Check sheet for the modelled part. Datum: model origin and axes. Units: mm. Face numbers are marked on the shaded views. A direction names the side the tool comes from. Round coordinates to 2 decimals unless told otherwise and drop trailing zeros. Order: outer loops, then holes, each group sorted by start corner. A loop starts at its lowest first (then second) coordinate and runs counter-clockwise, first axis right, second up.
Q1. Scan lines: probe 1 along X at (y, z) = (100, -7.5); probe 2 along X at (y, z) = (34, 19); probe 3 along Z at (x, y) = (-6, 18.5). Record each from-to range of solid material in increasing order.
Q2. Depth check by flat-ended pin: P1, Ø10, axis at x = 182, y = 97.5, coming from the +Z side; P2, Ø20, axis at x = 189.5, y = 98.5, coming from the -Z side; P3, Ø5, axis at y = 56.5, z = -30.5, coming from the +X side. Enter the tip coordinate at first touch or a pass-through.
Q3. Mould release check, pull along Z, two halves, no side actions. Record for the marked faces 6, 7 and 8: +Z half, -Z half, draft (parallel to the pull), parting line (faces both ways), or undercut.
Q4. Cross-section at C-C on z = -24.5. Record the cut outline in (x, y), then the cut area to 3 significant figures.
Q5. Cross-section at D-D on y = 112.5. Record the cut outline in (x, z).
Q6. Cross-section at B-B on y = 63.5. Record the cut outline in (x, z).
Q7. Set-up check for the marked faces 1, 2, 3, 4 and 5: record each of +Z, -Z, +X, -X, +Y, -Y from which the full face is reachable in a straight line by a thin tool's end or side.
Q8. Cross-section at A-A on x = -16. Record the cut outline in (y, z).
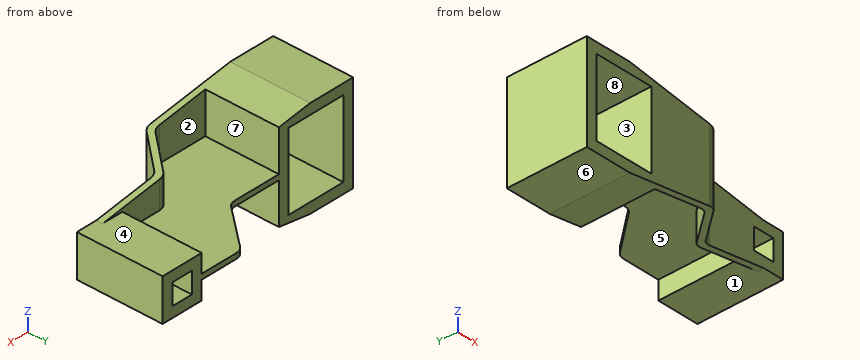
from build123d import *

# Parameters (mm, degrees)
SKIZZE1_W                       = 76
SKIZZE1_H                       = 93
AUFSATZ_LINEAR_AUSTRAGEN1_DEPTH = 76
AUFSATZ_LINEAR_AUSTRAGEN2_DEPTH = 46.5
SKIZZE3_W                       = 40
SKIZZE3_H                       = 40
AUFSATZ_LINEAR_AUSTRAGEN3_DEPTH = 81.5
AUFSATZ_LINEAR_AUSTRAGEN4_DEPTH = 2.5
SKIZZE5_W                       = 20
SKIZZE5_H                       = 20
SCHNITT_LINEAR_AUSTRAGEN1_DEPTH = 122.5
SKIZZE6_W                       = 56
SKIZZE6_H                       = 73
SCHNITT_LINEAR_AUSTRAGEN2_DEPTH = 77
SCHNITT_LINEAR_AUSTRAGEN3_DEPTH = 122.5
VERRUNDUNG1_R                   = 10


with BuildPart() as part:
    # Skizze1 → Aufsatz-Linear austragen1 (new body)
    with BuildSketch(Plane(origin=(0, 0, 0), x_dir=(1, 0, 0), z_dir=(0, 1, 0))):
        Rectangle(SKIZZE1_W, SKIZZE1_H)
    extrude(amount=AUFSATZ_LINEAR_AUSTRAGEN1_DEPTH)

    # Skizze2 → Aufsatz-Linear austragen2 (add, symmetric)
    with BuildSketch(Plane.XY):
        Polygon((38, 0), (92.436014753, 0), (126, 40), (186, 40), (186, 46), (123.202154051, 46), (89.638168804, 6), (38, 6), align=None)
    extrude(amount=AUFSATZ_LINEAR_AUSTRAGEN2_DEPTH, both=True)

    # Skizze3 → Aufsatz-Linear austragen3 (add)
    with BuildSketch(Plane.XZ.offset(-40)):
        with Locations((186, 0)):
            Rectangle(SKIZZE3_W, SKIZZE3_H)
    extrude(amount=-AUFSATZ_LINEAR_AUSTRAGEN3_DEPTH)

    # Skizze4 → Aufsatz-Linear austragen4 (add, symmetric)
    with BuildSketch(Plane.XY):
        Polygon((38, 76), (87.673704032, 76), (125.852737251, 121.5), (166, 121.5), (166, 46), (123.202154051, 46), (89.638168804, 6), (38, 6), align=None)
    extrude(amount=AUFSATZ_LINEAR_AUSTRAGEN4_DEPTH, both=True)

    # Skizze5 → Schnitt-Linear austragen1 (cut, through all)
    with BuildSketch(Plane(origin=(0, 121.5, 0), x_dir=(1, 0, 0), z_dir=(0, 1, 0))):
        with Locations((186, 0)):
            Rectangle(SKIZZE5_W, SKIZZE5_H)
    extrude(amount=-SCHNITT_LINEAR_AUSTRAGEN1_DEPTH, mode=Mode.SUBTRACT)

    # Skizze6 → Schnitt-Linear austragen2 (cut, through all)
    with BuildSketch(Plane(origin=(0, 76, 0), x_dir=(1, 0, 0), z_dir=(0, 1, 0))):
        Rectangle(SKIZZE6_W, SKIZZE6_H)
    extrude(amount=-SCHNITT_LINEAR_AUSTRAGEN2_DEPTH, mode=Mode.SUBTRACT)

    # Skizze7 → Schnitt-Linear austragen3 (cut, through all)
    with BuildSketch(Plane(origin=(0, 121.5, 0), x_dir=(1, 0, 0), z_dir=(0, 1, 0))):
        Polygon((6, 46.5), (186, 20), (186, 46.5), align=None)
        Polygon((6, -46.5), (186, -20), (186, -46.5), align=None)
    extrude(amount=-SCHNITT_LINEAR_AUSTRAGEN3_DEPTH, mode=Mode.SUBTRACT)

    # Verrundung1
    verrundung1_edges = [part.edges().sort_by_distance(p)[0] for p in [
        (126, 40, 0),
        (92.436014753, 0, 0),
        (89.638168804, 6, 18.343301463),
        (123.202154051, 46, 15.872619216),
        (89.638168804, 6, -18.343301463),
        (123.202154051, 46, -15.872619216),
        (125.852737251, 121.5, 0),
        (87.673704032, 76, 0),
    ]]
    fillet(verrundung1_edges, radius=VERRUNDUNG1_R)


solid = part.part
Results found:
1. probe 1: x = 166 to 176, 196 to 206
1. probe 2: x = -38 to -28, 28 to 38, 113.13 to 120.97
1. probe 3: z = -46.5 to -36.5, 36.5 to 46.5
2. P1: stops at z = 20
2. P2: stops at z = -20
2. P3: stops at x = 38
3. face 6: -Z half
3. face 7: draft
3. face 8: undercut
4. outline: (-38, 0) - (-28, 0) - (-28, 76) - (-38, 76) - close; (28, 0) - (87.77, 0) arc R10 ccw to (95.43, 3.57) - (123, 36.43) arc R10 cw to (130.66, 40) - (155.43, 40) - (155.43, 46) - (127.87, 46) arc R10 ccw to (120.2, 42.43) - (92.64, 9.57) arc R10 cw to (84.98, 6) - (38, 6) - (38, 76) - (28, 76) - close
4. area: 2,340 mm2
5. outline: (118.3, -2.5) - (166, -2.5) - (166, -20) - (206, -20) - (206, 20) - (166, 20) - (166, 2.5) - (118.3, 2.5) - close; hole (176, -10) - (196, -10) - (196, 10) - (176, 10) - close
6. outline: (-38, -46.5) - (6, -46.5) - (38, -41.79) - (38, -2.5) - (166, -2.5) - (166, -20) - (206, -20) - (206, 20) - (166, 20) - (166, 2.5) - (38, 2.5) - (38, 41.79) - (6, 46.5) - (-38, 46.5) - close; hole (-28, -36.5) - (28, -36.5) - (28, 36.5) - (-28, 36.5) - close; hole (176, -10) - (196, -10) - (196, 10) - (176, 10) - close
7. face 1: -Z, +X, +Y
7. face 2: +Z, +Y
7. face 3: +Y, -Y
7. face 4: +Z, +X, +Y
7. face 5: -Z, +Y
8. outline: (0, -46.5) - (76, -46.5) - (76, -36.5) - (0, -36.5) - close; (0, 36.5) - (76, 36.5) - (76, 46.5) - (0, 46.5) - close
